```python
from build123d import *

# Parameters (mm, degrees)
SKETCH1_R          = 5
BASE_EXTRUDE_DEPTH = 100
SKETCH5_OUTSIDE_W  = 32.2
SKETCH5_OUTSIDE_H  = 32.2
SKETCH5_OUTSIDE_R  = 3.5
FRONT_CUT_DEPTH    = 10
SKETCH2_R          = 1.5
FRONT_HOLE_DEPTH   = 10
CHAMFER1_SIZE      = 1
KEYWAY_CUT_DEPTH   = 15
SKETCH4_R          = 2
BACK_HOLE_DEPTH    = 20


with BuildPart() as part:
    # Sketch1 → Base Extrude (new body)
    with BuildSketch(Plane.XY):
        Circle(SKETCH1_R)
    extrude(amount=BASE_EXTRUDE_DEPTH)

    # Sketch5 outside → Front Cut (cut)
    with BuildSketch(Plane.XY.offset(100)):
        Rectangle(SKETCH5_OUTSIDE_W, SKETCH5_OUTSIDE_H)
        Circle(SKETCH5_OUTSIDE_R, mode=Mode.SUBTRACT)
    extrude(amount=-FRONT_CUT_DEPTH, mode=Mode.SUBTRACT)

    # Sketch2 → Front Hole (cut)
    with BuildSketch(Plane.XY.offset(100)):
        Circle(SKETCH2_R)
    extrude(amount=-FRONT_HOLE_DEPTH, mode=Mode.SUBTRACT)

    # Chamfer1
    chamfer1_edges = [part.edges().sort_by_distance(p)[0] for p in [
        (-3.5, 0, 100),
    ]]
    chamfer(chamfer1_edges, length=CHAMFER1_SIZE)

    # Sketch3 → Keyway Cut (cut)
    with BuildSketch(Plane.XY.offset(90)):
        with BuildLine():
            Line((4, 3), (4, -3))
            ThreePointArc((4, -3), (5, 0), (4, 3))
        make_face()
    extrude(amount=-KEYWAY_CUT_DEPTH, mode=Mode.SUBTRACT)

    # Sketch4 → Back Hole (cut)
    with BuildSketch(Plane(origin=(0, 0, 0), x_dir=(-1, 0, 0), z_dir=(0, 0, -1))):
        Circle(SKETCH4_R)
    extrude(amount=-BACK_HOLE_DEPTH, mode=Mode.SUBTRACT)


solid = part.part
```
Verification items for the finished model (mm, model axes). A direction names the side the tool comes from. Give positions to 0.01 mm unless a question says otherwise; leave off trailing zeros. Loops run counter-clockwise (first coordinate to the right, second up) from the corner with the lowest first, then second, coordinate; pieces in that order, holes last. Notation, with made-up numbers: M 55.25,71.25 L 109.25,71.25 A20 ccw 109.25,108.25 Z; hole C 46.25,41 d11. An arc over 180 degrees is marked long. Return JSON: item names as keys, results as strings.
1) Material ranges on L1, parallel to Y at x = 0, z = 94; L2, parallel to Y at x = 0, z = 7.5; L3, parallel to Z at x = -2.75, y = -3.25, recorded low to high. Write a range as [from, to].
Findings:
{"L1": "y = [-3.5, -1.5], [1.5, 3.5]", "L2": "y = [-5, -2], [2, 5]", "L3": "z = [0, 90]"}
2) Section check B-B, the plane x = 0. Enter the section's corners in (y, z).
Findings:
{"outline": "M -5,0 L -2,0 L -2,20 L 2,20 L 2,0 L 5,0 L 5,90 L 3.5,90 L 3.5,99 L 2.5,100 L 1.5,100 L 1.5,90 L -1.5,90 L -1.5,100 L -2.5,100 L -3.5,99 L -3.5,90 L -5,90 Z"}
3) Section check A-A, the plane y = 0. Enter the section's corners in (x, z), and give its area (3 significant figures).
Findings:
{"outline": "M -5,0 L -2,0 L -2,20 L 2,20 L 2,0 L 5,0 L 5,75 L 4,75 L 4,90 L 3.5,90 L 3.5,99 L 2.5,100 L 1.5,100 L 1.5,90 L -1.5,90 L -1.5,100 L -2.5,100 L -3.5,99 L -3.5,90 L -5,90 Z", "area": "844 mm2"}
4) Gauge pin test, flat ends, axial feed: P1, Ø2, axis at x = 0.5, y = 0, coming from the -Z side; P2, Ø1.8, axis at y = -1, z = 82, coming from the +X side; P3, Ø3, axis at x = -4, z = 14, coming from the -Y side; P4, Ø3.5, axis at x = 0, y = 0, coming from the +Z side. Record the tip position at first contact, or that the pin passes through.
Findings:
{"P1": "stops at z = 20", "P2": "stops at x = 4", "P3": "stops at y = -4.33", "P4": "stops at z = 100"}
5) Section check D-D, the plane z = 43. Enter the section's corners in (x, y).
Findings:
{"outline": "C 0,0 d10"}
6) Tool access check on faces 5 (the flat face through (4, 0, 83)), 6 (the flat face through (0, 0, 20)), 7 (the cylindrical face through (-5, 0, 44)), 8 (the flat face through (0, 0, 90)). Record the directions out of +Z, -Z, +X, -X, +Y, -Y that give a thin tool (end or side, any length) a straight path to the whole face; none if there is none.
Findings:
{"face 5": "+Z, +X, +Y, -Y", "face 6": "-Z", "face 7": "+Z, -Z", "face 8": "+Z"}
7) Mould release check, pull along X, two halves, no side actions. Record for faces 1 (the flat face through (-4, 0, 90)), 2 (the cylindrical face through (0, -2, 10)), 3 (the cylindrical face through (-1.5, 0.07, 95.07)), 4 (the cylindrical face through (3.233, -1.341, 94.563)): released by +X, released by -X, zero draft, split by the parting line, or undercut.
Findings:
{"face 1": "zero draft", "face 2": "undercut", "face 3": "undercut", "face 4": "split by the parting line"}
8) Section check C-C, the plane z = 17.5. Enter the section's corners in (x, y).
Findings:
{"outline": "C 0,0 d10; hole C 0,0 d4"}
